Source: CAD feature listing. Evaluate the final solid. Frame: model axes, mm. Give positions to 0.01 mm unless a question says otherwise; leave off trailing zeros. Order: outer loops, then holes, each group sorted by start corner. A loop starts at its lowest first (then second) coordinate and runs counter-clockwise, first axis right, second up.
1) Section B-B, the plane z = -117. Return loops of the section in (x, y), plus the area to 3 significant figures.
2) Section A-A, the plane y = 0.2. Return loops of the section in (x, z) (3 decimals), plus the area to 4 significant figures.
3) Section C-C, the plane z = -64.5. Return loops of the section in (x, y), plus the area to 3 significant figures.
4) Material intervals for line 1 (X direction, y = 0.35, z = -196); line 2 (X direction, y = 0.4, z = -168), sorted ascending.
```python
from build123d import *

# Parameters (mm, degrees)
BOSS_EXTRUDE1_DEPTH = 1
SKETCH2_W           = 14
SKETCH2_H           = 50
BOSS_EXTRUDE2_DEPTH = 1


with BuildPart() as part:
    # Sketch1 → Boss-Extrude1 (new body)
    with BuildSketch(Plane(origin=(0, 0, 0), x_dir=(1, 0, 0), z_dir=(0, 1, 0))):
        Polygon((9.725, 200), (4.275, 200), (0, 200), (4.275, 0), (9.725, 0), (14, 200), align=None)
    extrude(amount=BOSS_EXTRUDE1_DEPTH)

    # Sketch2 → Boss-Extrude2 (add)
    with BuildSketch(Plane.XZ):
        with Locations((7, -225)):
            Rectangle(SKETCH2_W, SKETCH2_H)
    extrude(amount=-BOSS_EXTRUDE2_DEPTH)


solid = part.part
```
From the geometry:
1. outline: (1.77, 0) - (12.23, 0) - (12.23, 1) - (1.77, 1) - close
1. area: 10.5 mm2
2. outline: (0, -250) - (14, -250) - (14, -200) - (9.725, 0) - (4.275, 0) - (0, -200) - close
2. area: 2,645 mm2
3. outline: (2.9, 0) - (11.1, 0) - (11.1, 1) - (2.9, 1) - close
3. area: 8.21 mm2
4. line 1: x = 0.09 to 13.91
4. line 2: x = 0.68 to 13.32
